Answer from the drawing. Dimensions are ordinates in mm from the lowest x, y and z of the part. A direction names the side the tool comes from. Give positions to 0.01 mm unless a question says otherwise; leave off trailing zeros. Loops run counter-clockwise (first coordinate to the right, second up) from the corner with the lowest first, then second, coordinate; pieces in that order, holes last. Notation, with made-up numbers: (-6.5, -35.5) - (6.5, -35.5) arc R28 cw to (6.5, -15.5) - close; hole circle Ø11 at (6, 39). An arc over 180 degrees is marked (long way). One line per item, written item: value.
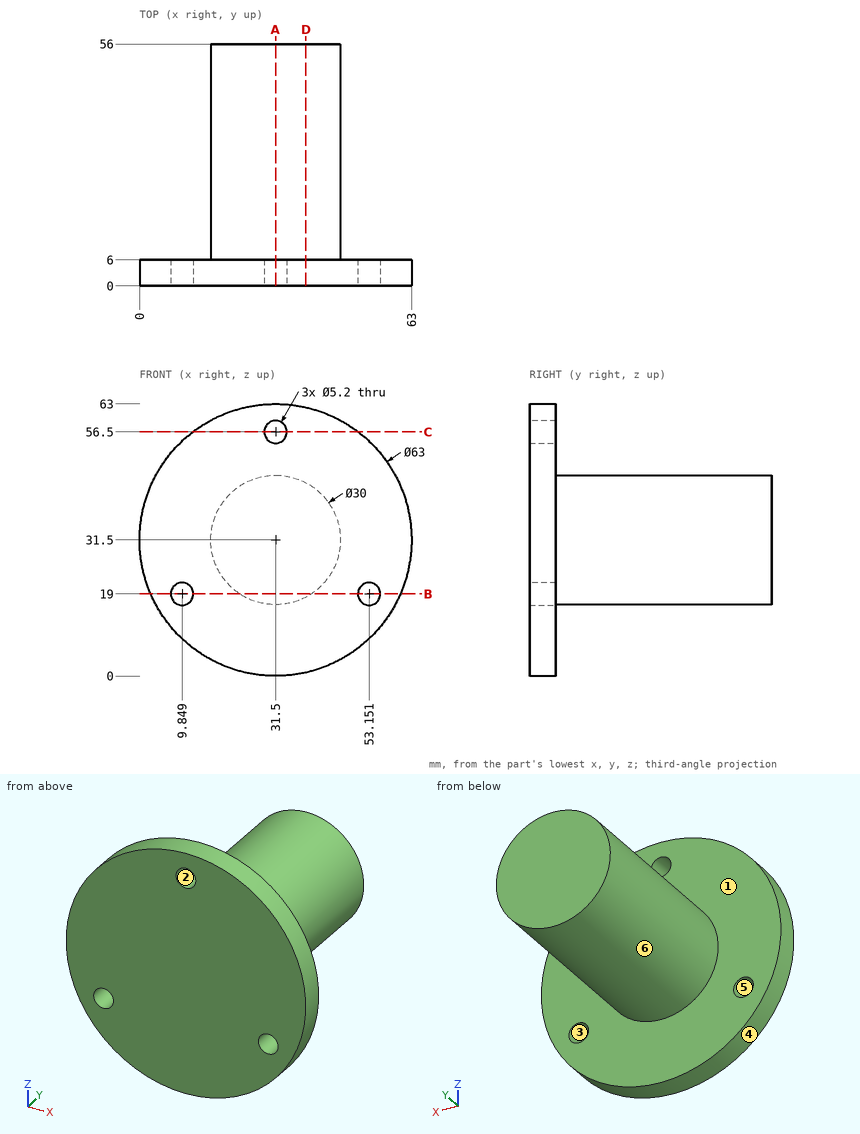
1. Section C-C (z = 56.5) is taken. Write down the section's boundary in (x, y).
Output:
outline: (12.34, 0) - (28.9, 0) - (28.9, 6) - (12.34, 6) - close; (34.1, 0) - (50.66, 0) - (50.66, 6) - (34.1, 6) - close
2. The mould has two halves that part along X. Classify the marked faces 1, 2, 3 and 4: released by +X, released by -X, zero draft, split by the parting line, or undercut.
Output:
face 1: zero draft
face 2: undercut
face 3: undercut
face 4: split by the parting line
3. Flat-ended cylindrical pins translate along their axes: pin 1 Ø3 at (y, z) = (15.5, 34) entering from +X; pin 2 Ø5 at (x, y) = (50.5, 15) entering from -Z; pin 3 Ø2 at (x, y) = (34, 23) entering from -Z (1 decimal); pin 4 Ø3 at (x, z) = (51.5, 31.5) entering from +Y. Find the tip coordinate at first contact, or state that the pin passes through.
Output:
pin 1: stops at x = 46.47
pin 2: passes through
pin 3: stops at z = 16.6
pin 4: stops at y = 6
4. Section D-D (x = 38.5) is taken. Write down the section's boundary in (y, z).
Output:
outline: (0, 0.79) - (6, 0.79) - (6, 18.23) - (56, 18.23) - (56, 44.77) - (6, 44.77) - (6, 62.21) - (0, 62.21) - close
5. Section A-A (x = 31.5) is taken. Write down the section's boundary in (y, z), and give its area (3 significant figures).
Output:
outline: (0, 0) - (6, 0) - (6, 16.5) - (56, 16.5) - (56, 46.5) - (6, 46.5) - (6, 53.9) - (0, 53.9) - close; (0, 59.1) - (6, 59.1) - (6, 63) - (0, 63) - close
area: 1,850 mm²
6. Find the intervals of material crossed by line 1 along X through (y, z) = (18, 31.5); line 2 along Y through (x, z) = (47, 45.5); line 3 along Z through (x, y) = (26.5, 49.5), in increasing order.
Output:
line 1: x = 16.5 to 46.5
line 2: y = 0 to 6
line 3: z = 17.36 to 45.64
7. For the marked faces 5 and 6, determine the directions among +Z, -Z, +X, -X, +Y, -Y from which every point of the face is accessible in a straight line to the end or side of a thin tool.
Output:
face 5: +Y, -Y
face 6: +Y
8. Section B-B (z = 19) is taken. Write down the section's boundary in (x, y).
Output:
outline: (2.59, 0) - (7.25, 0) - (7.25, 6) - (2.59, 6) - close; (12.45, 0) - (50.55, 0) - (50.55, 6) - (39.79, 6) - (39.79, 56) - (23.21, 56) - (23.21, 6) - (12.45, 6) - close; (55.75, 0) - (60.41, 0) - (60.41, 6) - (55.75, 6) - close
